For this review, take the finished solid that the model builds, in its own axes (mm). Face numbers are marked on the shaded views. A direction names the side the tool comes from. Round coordinates to 2 decimals unless told otherwise and drop trailing zeros. Write each loop counter-clockwise with the first axis right and the second up, starting at its lowest first coordinate (ties: lowest second). Pieces come first, ordered by that corner, then holes. Notation, with made-up numbers: M -36.75,49.5 L -9.75,49.5 A8 ccw -9.75,60.5 Z; hole C -9,-36.5 d8. An arc over 180 degrees is marked long. Write each question's results on one line, items separated by ' | '. Start each with the question number.
```python
from build123d import *

# Parameters (mm, degrees)
F0_W     = 108.235746
F0_H     = 80.899004
F1_DEPTH = 25.4
F3_DEPTH = 50.8


with BuildPart() as f1:
    # F0 (on Front) → F1 (new body)
    with BuildSketch(Plane.XZ):
        with Locations((0, -6.111877)):
            Rectangle(F0_W, F0_H)
    extrude(amount=-F1_DEPTH)

    # F2 (on face) → F3 (join)
    with BuildSketch(Plane.XZ):
        Polygon((-35.671126, -27.447874), (-54.117873, -27.447874), (-54.117873, -46.561379), (54.117873, -46.561379), (54.117873, -27.447874), (35.671126, -27.447874), align=None)
        Polygon((-54.117873, 0), (-54.117873, -27.447874), (-35.671126, -27.447874), align=None)
        Polygon((54.117873, 0), (35.671126, -27.447874), (54.117873, -27.447874), align=None)
    extrude(amount=F3_DEPTH)


solid = f1.part
```
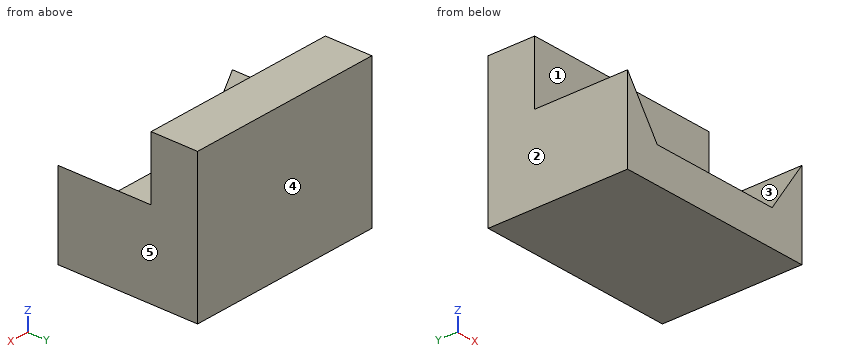
Item 1: For the marked faces 1 and 2, list the 3-axis set-ups (+Z, -Z, +X, -X, +Y, -Y) from which the entire face can be reached by the end or side of a thin tool; tool diameter is ignored.
Item 2: We need section C-C on y = -7. State the section outline as (x, z) points.
Item 3: We need section A-A on z = 6. State the section outline as (x, y) points.
Item 4: Mouldability with a two-part tool opening along X and no side actions: class the marked faces 3, 4 and 5 as pulls with the +X half, pulls with the -X half, needs draft (parallel to the pull), parting line crosses it, or undercut.
Item 5: We need section B-B on x = 13. State the section outline as (y, z) points.
Item 6: For probe 1 along Z at (x, y) = (-16, -21); probe 2 along Y at (x, z) = (-11.5, -1); probe 3 along X at (y, z) = (-12, -10), list the stretches that pass through material, from the lowest coordinate up.
Numbers:
1) face 1: +Z, -Y | face 2: +Z, -Z, -X, +Y, -Y
2) outline: M -54.12,-46.56 L 54.12,-46.56 L 54.12,0 L 35.67,-27.45 L -35.67,-27.45 L -54.12,0 Z
3) outline: M -54.12,0 L 54.12,0 L 54.12,25.4 L -54.12,25.4 Z
4) face 3: undercut | face 4: needs draft | face 5: pulls with the +X half
5) outline: M -50.8,-46.56 L 25.4,-46.56 L 25.4,34.34 L 0,34.34 L 0,-27.45 L -50.8,-27.45 Z
6) probe 1: z = -46.56 to -27.45 | probe 2: y = 0 to 25.4 | probe 3: x = -54.12 to -47.4, 47.4 to 54.12
